Could you check a few things on this model? Use its own coordinates, in mm. A direction names the side the tool comes from. Coordinates: 2 decimals unless noted, no trailing zeros. Write each loop counter-clockwise with the first axis right and the second up, starting at its lowest first coordinate (ties: lowest second). Pieces come first, ordered by that corner, then holes. Notation, with made-up numbers: M 60.5,68.25 L 89.5,68.25 A16 ccw 89.5,99.25 Z; hole C 43,44.5 d1. An arc over 180 degrees is marked long. Write item = value, one per line.
```python
from build123d import *

# Parameters (mm, degrees)
SKETCH2_OUTSIDE_W  = 25.78
SKETCH2_OUTSIDE_H  = 25.78
CUT_EXTRUDE1_DEPTH = 27.994890987


with BuildPart() as part:
    # Sketch1 → Revolve1 (revolve)
    with BuildSketch(Plane(origin=(0, 0, 0), x_dir=(0, 0, -1), z_dir=(1, 0, 0)), mode=Mode.PRIVATE) as revolve1_sk:
        Polygon((-4.127129718, 2.3876), (-24.591144492, 2.3876), (-24.591144492, 2.936534554), (-21.543144492, 3.2032), (-21.523850338, 2.982666814), (-19.003144492, 3.2032), (-18.985366795, 3), (-5.541144492, 3), (-5.541144492, 5.334), (-4.616660097, 7.874), (-0.924484395, 7.874), (0, 5.334), (0, 5.1562), (8.825478894, 4.539062397), (8.825478894, 2.5781), (-4.017144492, 2.5781), align=None)
    revolve(revolve1_sk.sketch.rotate(Axis((0, 0, -2.001994087), (0, 0, -1)), 90), axis=Axis((0, 0, -2.001994087), (0, 0, -1)))

    # Sketch2 outside → Cut-Extrude1 (cut, through all)
    with BuildSketch(Plane.XY):
        Rectangle(SKETCH2_OUTSIDE_W, SKETCH2_OUTSIDE_H)
        Polygon((0, 6.423137215), (-5.5626, 3.211568607), (-5.5626, -3.211568607), (0, -6.423137215), (5.5626, -3.211568607), (5.5626, 3.211568607), align=None, mode=Mode.SUBTRACT)
    extrude(amount=CUT_EXTRUDE1_DEPTH, mode=Mode.SUBTRACT)


solid = part.part
```
Item 1: If we mould it in two halves opening along Y, with no side actions, what happens to faces 1 (the face through (-2.82, -4.795, 2.733)), 2 (the face through (-3.84, 2.95, -4.47)), 3 (the face through (-0.52, 2.33, 14.5))? For each: pulls with the +Y half, pulls with the -Y half, needs draft (parallel to the pull), parting line crosses it, or undercut.
Numbers:
face_1 = pulls with the -Y half
face_2 = parting line crosses it
face_3 = undercut
Item 2: I'm going to push flat-ended pins straight in: P1, Ø5, axis at x = -4, z = -5.5, coming from the -Y side; P2, Ø5.5, axis at x = 0, y = 0, coming from the -Z side; P3, Ø2, axis at x = -3.5, z = -3, coming from the +Y side; P4, Ø1, axis at y = -0.5, z = 16.5, coming from the -X side. Where does each tip first touch, or does it pass through?
Numbers:
P1 = -4.55
P2 = -8.83
P3 = 4.27
P4 = -3
Item 3: Imagine slicing it at B-B (z = 18.5). Write out the boundary of the cut face in (x, y).
Numbers:
outline = C 0,0 d6; hole C 0,0 d4.78
Item 4: If I drill on line 1 along Y through (x, z) = (0, 12.5); line 2 along Z through (x, y) = (-2.25, 3.5); line 3 along Y through (x, z) = (0, -1.25), over which ranges is the centre line in solid material (lowest first)?
Numbers:
line_1 = -3 to -2.39, 2.39 to 3
line_2 = -8.83 to 5.54
line_3 = -5.07 to -2.58, 2.58 to 5.07
Item 5: For faces 4 (the face through (-0.336, -2.556, -2.314)), 5 (the face through (5.563, 0, 3)), 6 (the face through (2.86, -0.9, 12.17)), which set-ups out of +Z, -Z, +X, -X, +Y, -Y let a thin tool reach every point of the face, with its end or its side?
Numbers:
face_4 = -Z
face_5 = +Z, -Z, +X, +Y, -Y
face_6 = none
